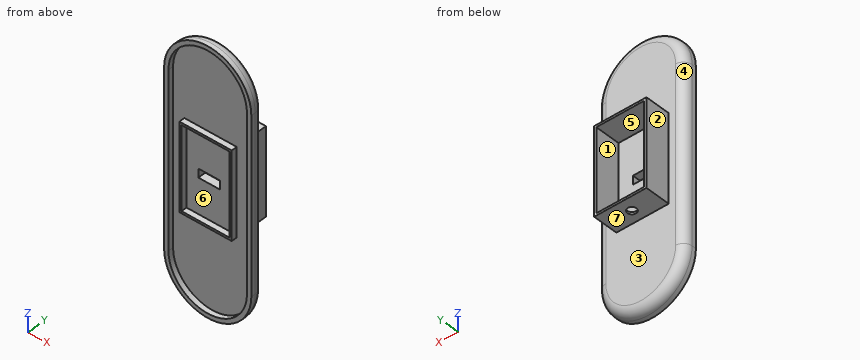
```python
from build123d import *

# Parameters (mm, degrees)
ESQUISSE1_R                  = 50
ESQUISSE1_W                  = 100
ESQUISSE1_H                  = 200
BOSS_EXTRU_2_DEPTH           = 15
CONG_3_R                     = 10
ESQUISSE1_5_W                = 90
ESQUISSE1_5_H                = 200
ENL_V_MAT_EXTRU_6_DEPTH      = 6
BOSS_EXTRU_3_DEPTH           = 44
BOSS_EXTRU_3_DEPTH_BACK      = 0.5
ESQUISSE1_6_W                = 60
ESQUISSE1_6_H                = 100
ESQUISSE1_6_W_2              = 55
ESQUISSE1_6_H_2              = 95
ENL_V_MAT_EXTRU_7_DEPTH      = 90
ENL_V_MAT_EXTRU_7_DEPTH_BACK = 131
ESQUISSE1_10_W               = 25
ESQUISSE1_10_H               = 10
ESQUISSE6_R                  = 5.118807206
ENL_V_MAT_EXTRU_8_DEPTH      = 13


with BuildPart() as part:
    # Esquisse1 → Boss.-Extru.2 (new body)
    with BuildSketch(Plane(origin=(0, 0, 0), x_dir=(1, 0, 0), z_dir=(0, 1, 0))):
        with Locations((-0.858369099, 46.305967004)):
            Circle(ESQUISSE1_R)
        with Locations((-0.858369099, -153.694032996)):
            Circle(ESQUISSE1_R)
        with Locations((-0.858369099, -53.694032996)):
            Rectangle(ESQUISSE1_W, ESQUISSE1_H)
    extrude(amount=BOSS_EXTRU_2_DEPTH)

    # Cong_3
    cong_3_edges = [part.edges().sort_by_distance(p)[0] for p in [
        (-50.858369099, 15, 53.694032996),
        (49.141630901, 15, 53.694032996),
        (-0.858369099, 15, 203.694032996),
        (-0.858369099, 15, -96.305967004),
    ]]
    fillet(cong_3_edges, radius=CONG_3_R)

    # Esquisse1_5 → Enl_v. mat.-Extru.6 (cut)
    with BuildSketch(Plane(origin=(0, 0, 0), x_dir=(1, 0, 0), z_dir=(0, 1, 0))):
        with BuildLine():
            ThreePointArc((44.141630901, 46.305967004), (-0.858369099, 91.305967004), (-45.858369099, 46.305967004))
            Line((-45.858369099, 46.305967004), (44.141630901, 46.305967004))
        make_face()
        with BuildLine():
            Line((44.141630901, 46.305967004), (-45.858369099, 46.305967004))
            ThreePointArc((-45.858369099, 46.305967004), (-0.858369099, 1.305967004), (44.141630901, 46.305967004))
        make_face()
        with BuildLine():
            ThreePointArc((44.141630901, -153.694032996), (-0.858369099, -108.694032996), (-45.858369099, -153.694032996))
            Line((-45.858369099, -153.694032996), (44.141630901, -153.694032996))
        make_face()
        with BuildLine():
            Line((44.141630901, -153.694032996), (-45.858369099, -153.694032996))
            ThreePointArc((-45.858369099, -153.694032996), (-0.858369099, -198.694032996), (44.141630901, -153.694032996))
        make_face()
        with Locations((-0.858369099, -53.694032996)):
            Rectangle(ESQUISSE1_5_W, ESQUISSE1_5_H)
    extrude(amount=ENL_V_MAT_EXTRU_6_DEPTH, mode=Mode.SUBTRACT)

    # Esquisse1_6 → Boss.-Extru.3 (add, two sides: drawn at the far end of the back side and taken through both)
    with BuildSketch(Plane(origin=(0, 0, 0), x_dir=(1, 0, 0), z_dir=(0, 1, 0)).offset(-BOSS_EXTRU_3_DEPTH_BACK)):
        with Locations((-2.915547204, -53.694032996)):
            Rectangle(ESQUISSE1_6_W, ESQUISSE1_6_H)
        with Locations((-2.915547204, -53.694032996)):
            Rectangle(ESQUISSE1_6_W_2, ESQUISSE1_6_H_2, mode=Mode.SUBTRACT)
    extrude(amount=BOSS_EXTRU_3_DEPTH + BOSS_EXTRU_3_DEPTH_BACK)

    # Esquisse1_10 → Enl_v. mat.-Extru.7 (cut, two sides: drawn at the far end of the back side and taken through both)
    with BuildSketch(Plane(origin=(0, 0, 0), x_dir=(1, 0, 0), z_dir=(0, 1, 0)).offset(-ENL_V_MAT_EXTRU_7_DEPTH_BACK)):
        with Locations((-4.32906887, -51.451666969)):
            Rectangle(ESQUISSE1_10_W, ESQUISSE1_10_H)
    extrude(amount=ENL_V_MAT_EXTRU_7_DEPTH + ENL_V_MAT_EXTRU_7_DEPTH_BACK, mode=Mode.SUBTRACT)

    # Esquisse6 → Enl_v. mat.-Extru.8 (cut)
    with BuildSketch(Plane.XY):
        with Locations(Location((-2.915547204, 28.813279857, 0), (0, 0, 180))):
            Circle(ESQUISSE6_R)
    extrude(amount=ENL_V_MAT_EXTRU_8_DEPTH, mode=Mode.SUBTRACT)


solid = part.part
```
Can you work these out from the model? Positions are in its coordinate system, mm. Face numbers are marked on the shaded views. A direction names the side the tool comes from. Give positions to 0.01 mm unless a question says otherwise; leave off trailing zeros. Order: outer loops, then holes, each group sorted by start corner. A loop starts at its lowest first (then second) coordinate and runs counter-clockwise, first axis right, second up. Notation, with made-up numbers: M 76.25,8.5 L 111.25,8.5 A28 cw 111.25,27.5 Z; hole C 60,73 d4. An arc over 180 degrees is marked long. Write item = value, one per line. Start each with the question number.
Q1. Suppose I cut it at A-A (y = 37). Write out the boundary of the cut face in (x, z).
Q2. I need wall thicknesses on probe 1 along X at (y, z) = (3.5, 122.5); probe 2 along Z at (x, y) = (10.5, 18.5); probe 3 along Y at (x, z) = (-11, -75). Which ranges of each line are inside material? Lowest first, please. Write a range as [from, to].
Q3. For the marked faces 4, 5, 6 and 7, which set-ups out of +Z, -Z, +X, -X, +Y, -Y let a thin tool reach every point of the face, with its end or its side?
Q4. Suppose I cut it at C-C (x = -2.5). Count the separate pieces of the cut face and the enclosed holes in it, plus the area to 3 significant figures.
Q5. Suppose I cut it at B-B (z = -36.5). Write out the boundary of the cut face in (x, y).
Q6. We'd pull the mould along X, two halves only. Please class the marked faces 1, 2 and 3: pulls with the +X half, pulls with the -X half, needs draft (parallel to the pull), parting line crosses it, or undercut.
Q7. Will these pins go through, and if not, where does the flat tip stop? pin 1 Ø14.5 at (y, z) = (35, 50.5) entering from +X; pin 2 Ø5 at (x, y) = (-4, 1.5) entering from -Z; pin 3 Ø4 at (x, z) = (15.5, 58.5) entering from -Y.
Check result:
q1.outline = M -32.92,3.69 L 27.08,3.69 L 27.08,103.69 L -32.92,103.69 Z; hole M -30.42,6.19 L 24.58,6.19 L 24.58,101.19 L -30.42,101.19 Z
q2.probe_1 = [-50.86, -45.86], [44.14, 49.14]
q2.probe_2 = [3.69, 6.19], [101.19, 103.69]
q2.probe_3 = [6, 15]
q3.face_4 = +Z, -Z, -X, +Y
q3.face_5 = +Y
q3.face_6 = -Y
q3.face_7 = -Z, +X, -X, +Y
q4.separate_pieces = 3
q4.enclosed_holes = 0
q4.area = 2,780 mm2
q5.outline = M -50.86,0 L -45.86,0 L -45.86,6 L 44.14,6 L 44.14,0 L 49.14,0 L 49.14,5 A10 ccw 39.14,15 L -40.86,15 A10 ccw -50.86,5 Z
q6.face_1 = undercut
q6.face_2 = pulls with the -X half
q6.face_3 = needs draft
q7.pin_1 = 27.08
q7.pin_2 = -96.3
q7.pin_3 = 6
